```python
from build123d import *

# Parameters (mm, degrees)
ESBO_O1_W             = 27
ESBO_O1_H             = 22
ESBO_O1_W_2           = 25
ESBO_O1_H_2           = 20
EXTRUS_O_FINA1_DEPTH  = 20
ESBO_O2_R             = 5
CORTE_EXTRUS_O1_DEPTH = 23
ESBO_O3_R             = 2
CORTE_EXTRUS_O2_DEPTH = 10


with BuildPart() as part:
    # Esboço1 → Extrusão-Fina1 (new body)
    with BuildSketch(Plane.XY):
        with Locations((-12.5, 10)):
            Rectangle(ESBO_O1_W, ESBO_O1_H)
        with Locations((-12.5, 10)):
            Rectangle(ESBO_O1_W_2, ESBO_O1_H_2, mode=Mode.SUBTRACT)
    extrude(amount=EXTRUS_O_FINA1_DEPTH)

    # Esboço2 → Corte-extrusão1 (cut, through all)
    with BuildSketch(Plane(origin=(0, 21, 0), x_dir=(1, 0, 0), z_dir=(0, 1, 0))):
        with Locations(Location((-16.944433868, -12.551828058, 0), (0, 0, 180))):  # turned: the seam where the file's is
            Circle(ESBO_O2_R)
    extrude(amount=-CORTE_EXTRUS_O1_DEPTH, mode=Mode.SUBTRACT)

    # Esboço3 → Corte-extrusão2 (cut)
    with BuildSketch(Plane(origin=(0, 21, 0), x_dir=(1, 0, 0), z_dir=(0, 1, 0))):
        with Locations(Location((-2.78489643, -15.508719635, 0), (0, 0, 180))):  # turned: the seam where the file's is
            Circle(ESBO_O3_R)
    extrude(amount=-CORTE_EXTRUS_O2_DEPTH, mode=Mode.SUBTRACT)


solid = part.part
```
Part model, mm, in its own coordinate system. A direction names the side the tool comes from. Round coordinates to 2 decimals unless told otherwise and drop trailing zeros. Order: outer loops, then holes, each group sorted by start corner. A loop starts at its lowest first (then second) coordinate and runs counter-clockwise, first axis right, second up. Notation, with made-up numbers: M -25,5.25 L 23,5.25 A24 cw 23,34.25 Z; hole C 76,-9 d6. An arc over 180 degrees is marked long. Put each result on its own line as item: value. Start each with the question number.
1. Slice it at D-D on z = 11. List the corners of the cut face in (x, y).
2. Slice it at C-C on z = 19.25. List the corners of the cut face in (x, y).
3. Two-plate mould, pull along Z, no slides. Class faces 1 (the face through (-13, 20, 8)), 2 (the face through (-13.6, -0.5, 20)), 3 (the face through (-15.86, -0.49, 7.67)), 4 (the face through (-3.86, 20.507, 17.195)): +Z half, -Z half, draft (parallel to the pull), parting line (faces both ways), or undercut.
4. Drill centre lines: probe 1 along Y at (x, z) = (-5.5, 11); probe 2 along X at (y, z) = (14.25, 15.25); probe 3 along Y at (x, z) = (-2.5, 17). Where is each one in solid material? Low to high. Write a range as [from, to].
5. Tool access for faces 5 (the face through (-15.86, 20.51, 7.67)), 6 (the face through (0, 10, 10)): list every direction of +Z, -Z, +X, -X, +Y, -Y with a clear straight run to the whole face (end or side of a thin tool).
6. Slice it at A-A on x = -6. List the corners of the cut face in (y, z), then the cut area to 3 significant figures.
7. Slice it at B-B on y = 19.25. List the corners of the cut face in (x, z), then the cut area to 3 significant figures.
Findings:
1. outline: M -26,-1 L -21.7,-1 L -21.7,0 L -25,0 L -25,20 L -21.7,20 L -21.7,21 L -26,21 Z; M -12.19,-1 L 1,-1 L 1,21 L -12.19,21 L -12.19,20 L 0,20 L 0,0 L -12.19,0 Z
2. outline: M -26,-1 L 1,-1 L 1,21 L -26,21 Z; hole M -25,0 L 0,0 L 0,20 L -25,20 Z
3. face 1: draft
3. face 2: +Z half
3. face 3: undercut
3. face 4: undercut
4. probe 1: [-1, 0], [20, 21]
4. probe 2: [-26, -25], [0, 1]
4. probe 3: [-1, 0]
5. face 5: +Y, -Y
5. face 6: +Z, -Z
6. outline: M -1,0 L 0,0 L 0,20 L -1,20 Z; M 20,0 L 21,0 L 21,20 L 20,20 Z
6. area: 40.0 mm2
7. outline: M -26,0 L -25,0 L -25,20 L -26,20 Z; M 0,0 L 1,0 L 1,20 L 0,20 Z
7. area: 40.0 mm2
